For this review, use the dimensioned drawing (mm, ordinates from the lowest corner) and the shaded views. A direction names the side the tool comes from. Give positions to 0.01 mm unless a question says otherwise; leave off trailing zeros. Loops run counter-clockwise (first coordinate to the right, second up) from the corner with the lowest first, then second, coordinate; pieces in that order, holes last. Notation, with made-up numbers: M -10,3.25 L 33,3.25 A26 ccw 33,28.25 Z; hole C 9.5,-9.75 d10. An arc over 180 degrees is marked long. Return JSON: item names as keys, results as strings.
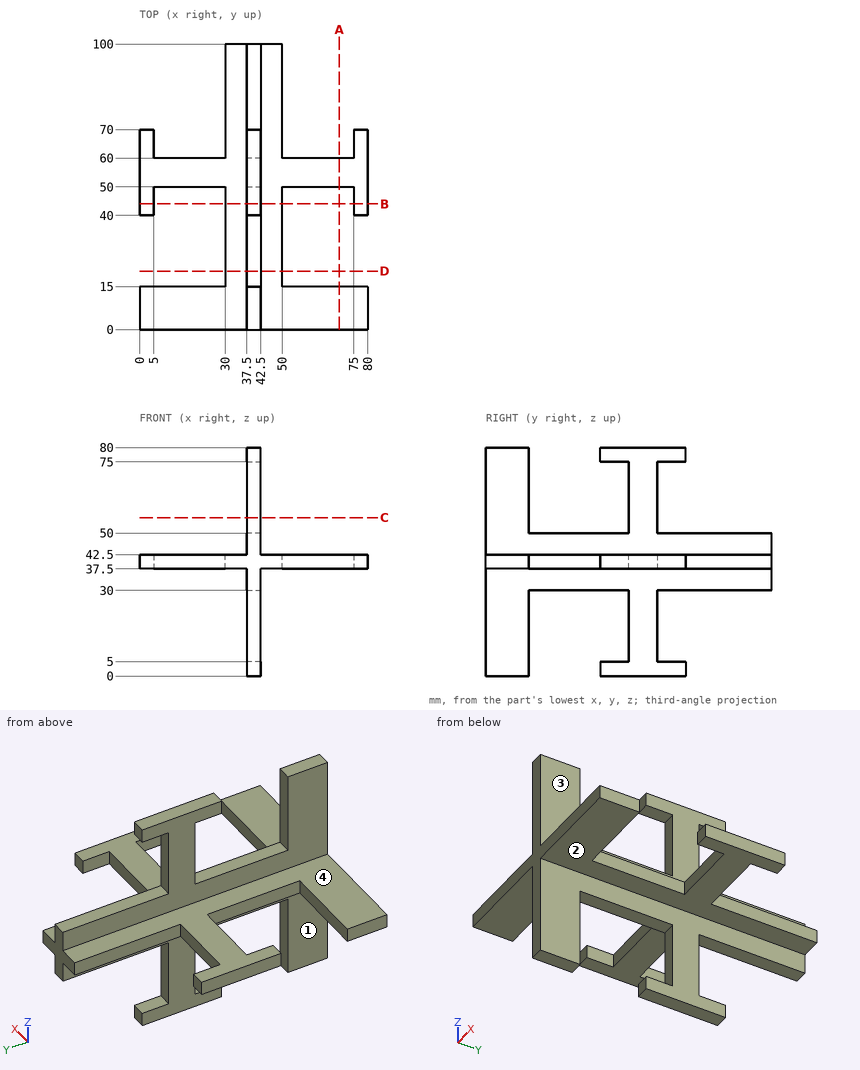
1) Consider section A-A on x = 70. Write out the cut boundary in (y, z), then the cut area to 3 significant figures.
From the geometry:
{"outline": "M 0,37.5 L 15,37.5 L 15,42.5 L 0,42.5 Z; M 50,37.5 L 60,37.5 L 60,42.5 L 50,42.5 Z", "area": "125 mm²"}
2) Consider section C-C on z = 55.5. Write out the cut boundary in (x, y).
From the geometry:
{"outline": "M 37.5,0 L 42.5,0 L 42.5,15 L 37.5,15 Z; M 37.5,50 L 42.5,50 L 42.5,60 L 37.5,60 Z"}
3) Wall thickness on L1, parallel to Z at x = 38, y = 65.5; L2, parallel to Y at x = 9.5, z = 38.5; L3, parallel to Z at x = 46, y = 16: over which ranges is each line inside the solid? List them lowest first. Write a range as from..to.
From the geometry:
{"L1": "0..5, 30..50, 75..80", "L2": "0..15, 50..60", "L3": "37.5..42.5"}
4) Tool access review of the marked faces 1, 2, 3 and 4: name each direction out of +Z, -Z, +X, -X, +Y, -Y from which nothing blocks a thin tool from reaching the whole face with its end or side.
From the geometry:
{"face 1": "-Z, -X, +Y, -Y", "face 2": "-Z, +X, +Y, -Y", "face 3": "+Z, +X, +Y, -Y", "face 4": "+Z, -X, +Y, -Y"}
5) Consider section D-D on y = 20.5. Write out the cut boundary in (x, z), then the cut area to 3 significant figures.
From the geometry:
{"outline": "M 30,37.5 L 37.5,37.5 L 37.5,30 L 42.5,30 L 42.5,37.5 L 50,37.5 L 50,42.5 L 42.5,42.5 L 42.5,50 L 37.5,50 L 37.5,42.5 L 30,42.5 Z", "area": "175 mm²"}
6) Insertion check: pin 1 (8 mm diameter, centred on y = 52, z = 25, fed in from +X); pin 2 (2.5 mm diameter, centred on x = 15.5, z = 40, fed in from +Y); pin 3 (5.5 mm diameter, centred on y = 75.5, z = 39, fed in from -X). Each pin has a flat end and moves straight along its axis. Give the tip position at first contact, or say it passes through.
From the geometry:
{"pin 1": "x = 42.5", "pin 2": "y = 60", "pin 3": "x = 30"}
7) Consider section B-B on y = 44. Write out the cut boundary in (x, z), then the cut area to 3 significant figures.
From the geometry:
{"outline": "M 0,37.5 L 5,37.5 L 5,42.5 L 0,42.5 Z; M 30,37.5 L 37.5,37.5 L 37.5,30 L 42.5,30 L 42.5,37.5 L 50,37.5 L 50,42.5 L 42.5,42.5 L 42.5,50 L 37.5,50 L 37.5,42.5 L 30,42.5 Z; M 37.5,0 L 42.5,0 L 42.5,5 L 37.5,5 Z; M 37.5,75 L 42.5,75 L 42.5,80 L 37.5,80 Z; M 75,37.5 L 80,37.5 L 80,42.5 L 75,42.5 Z", "area": "275 mm²"}
